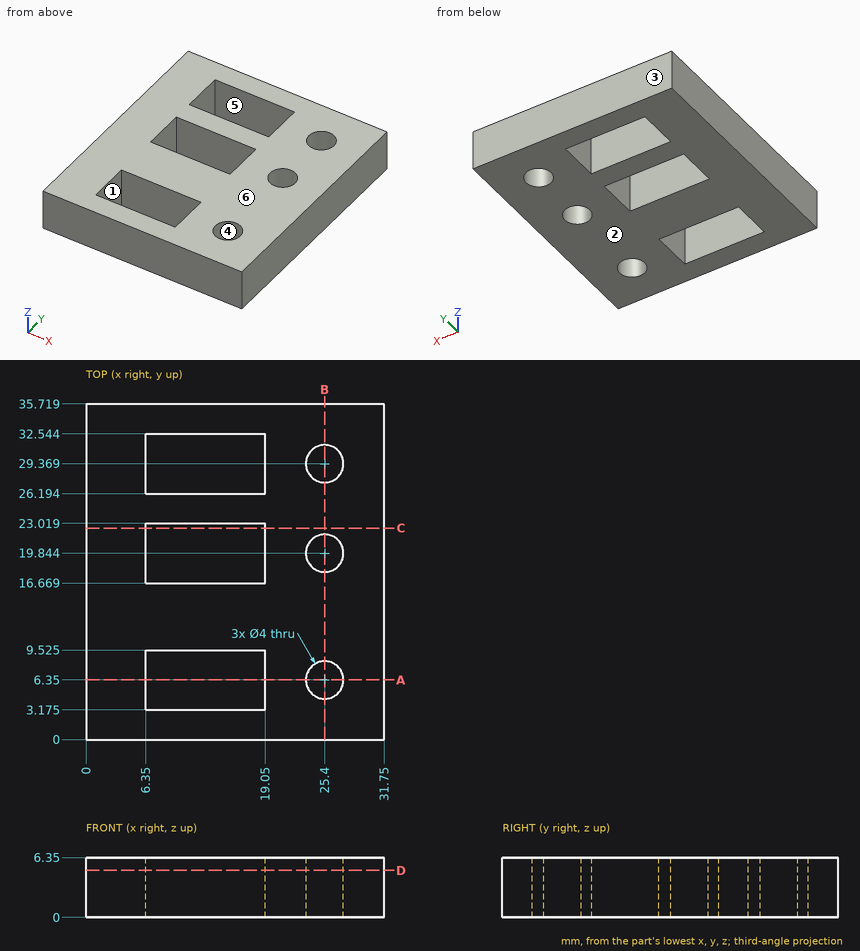
Could you check a few things on this drawing? It's one solid part, dimensions in mm from its lowest x, y, z. A direction names the side the tool comes from. Coordinates: 2 decimals unless noted, no trailing zeros. Write each loop counter-clockwise with the first axis right and the second up, starting at its lowest first coordinate (ties: lowest second). Pieces come first, ordered by that corner, then holes.
Q1. Imagine slicing it at A-A, the plane y = 6.35. List the corners of the cut face in (x, z) for me.
Results found:
outline: (0, 0) - (6.35, 0) - (6.35, 6.35) - (0, 6.35) - close; (19.05, 0) - (23.4, 0) - (23.4, 6.35) - (19.05, 6.35) - close; (27.4, 0) - (31.75, 0) - (31.75, 6.35) - (27.4, 6.35) - close
Q2. For P1, Ø6.5, axis at x = 25.4, y = 19.84, coming from the +Z side; P2, Ø3, axis at x = 25.4, y = 29.37, coming from the -Z side, each with a flat end and sliding along its axis, tell me the tip position at first contact or that it passes through.
Results found:
P1: stops at z = 6.35
P2: passes through
Q3. Imagine slicing it at B-B, the plane x = 25.4. List the corners of the cut face in (y, z) for me.
Results found:
outline: (0, 0) - (4.35, 0) - (4.35, 6.35) - (0, 6.35) - close; (8.35, 0) - (17.84, 0) - (17.84, 6.35) - (8.35, 6.35) - close; (21.84, 0) - (27.37, 0) - (27.37, 6.35) - (21.84, 6.35) - close; (31.37, 0) - (35.72, 0) - (35.72, 6.35) - (31.37, 6.35) - close
Q4. If we mould it in two halves opening along Y, with no side actions, what happens to the marked faces 1, 2, 3 and 4? For each: +Y half, -Y half, draft (parallel to the pull), parting line (faces both ways), or undercut.
Results found:
face 1: undercut
face 2: draft
face 3: +Y half
face 4: undercut
Q5. Imagine slicing it at C-C, the plane y = 22.5. List the corners of the cut face in (x, z) for me.
Results found:
outline: (0, 0) - (6.35, 0) - (6.35, 6.35) - (0, 6.35) - close; (19.05, 0) - (31.75, 0) - (31.75, 6.35) - (19.05, 6.35) - close
Q6. Imagine slicing it at D-D, the plane z = 5. Count the separate pieces of the cut face and the enclosed holes in it.
Results found:
separate pieces: 1
enclosed holes: 6
Q7. Which directions (+Z, -Z, +X, -X, +Y, -Y) give clear straight access to the entire face, cutting with the end or side of a thin tool? Please do the marked faces 5 and 6.
Results found:
face 5: +Z, -Z
face 6: +Z, +X, -X, +Y, -Y
Q8. Please list where these lines run through material, in increasing order: L1, parallel to Y at x = 25.4, z = 1.5; L2, parallel to X at y = 20, z = 2; L3, parallel to X at y = 3.5, z = 2.5.
Results found:
L1: y = 0 to 4.35, 8.35 to 17.84, 21.84 to 27.37, 31.37 to 35.72
L2: x = 0 to 6.35, 19.05 to 23.41, 27.39 to 31.75
L3: x = 0 to 6.35, 19.05 to 31.75
